Read the model definition and answer for the solid it produces. Units are mm, in the model's axes. A direction names the side the tool comes from. Coordinates: 2 decimals unless noted, no trailing zeros. Order: outer loops, then holes, each group sorted by start corner. A loop starts at its lowest first (then second) coordinate and runs counter-clockwise, first axis right, second up. Notation, with made-up numbers: (52, 52.5) - (85, 52.5) arc R24 ccw to (85, 79.5) - close; hole circle Ø3 at (24, -15.5). An arc over 180 degrees is marked (long way). Use one line per item in the form item = value.
```python
from build123d import *

# Parameters (mm, degrees)
ESBO_O1_W                = 100
ESBO_O1_H                = 100
RESSALTO_EXTRUS_O1_DEPTH = 5
ESBO_O2_R                = 7.5
ESBO_O2_R_2              = 5
RESSALTO_EXTRUS_O2_DEPTH = 60


with BuildPart() as part:
    # Esboço1 → Ressalto-extrusão1 (new body)
    with BuildSketch(Plane(origin=(0, 0, 0), x_dir=(1, 0, 0), z_dir=(0, 1, 0))):
        Rectangle(ESBO_O1_W, ESBO_O1_H)
    extrude(amount=-RESSALTO_EXTRUS_O1_DEPTH)

    # Esboço2 → Ressalto-extrusão2 (add)
    with BuildSketch(Plane(origin=(0, 0, 0), x_dir=(1, 0, 0), z_dir=(0, 1, 0))):
        with Locations(Location((0, 0, 0), (0, 0, 270))):
            Circle(ESBO_O2_R)
        with Locations(Location((0, 0, 0), (0, 0, 270))):
            Circle(ESBO_O2_R_2, mode=Mode.SUBTRACT)
    extrude(amount=RESSALTO_EXTRUS_O2_DEPTH)


solid = part.part
```
(1) Section A-A, the plane z = 0 is taken. Write down the section's boundary in (x, y).
Answer list:
outline = (-50, -5) - (50, -5) - (50, 0) - (7.5, 0) - (7.5, 60) - (5, 60) - (5, 0) - (-5, 0) - (-5, 60) - (-7.5, 60) - (-7.5, 0) - (-50, 0) - close
(2) Section D-D, the plane z = -15 is taken. Write down the section's boundary in (x, y), then the cut area to 3 significant figures.
Answer list:
outline = (-50, -5) - (50, -5) - (50, 0) - (-50, 0) - close
area = 500 mm2
(3) Given pin 1 Ø5 at (x, z) = (10.5, 10.5) entering from +Y; pin 2 Ø6 at (x, y) = (0.5, 43.5) entering from -Z, each flat-ended and moving along its own axis, determine where each tip first touches the part or whether it passes through.
Answer list:
pin_1 = 0
pin_2 = -7.5
(4) Section B-B, the plane x = 0 is taken. Write down the section's boundary in (y, z).
Answer list:
outline = (-5, -50) - (0, -50) - (0, -7.5) - (60, -7.5) - (60, -5) - (0, -5) - (0, 5) - (60, 5) - (60, 7.5) - (0, 7.5) - (0, 50) - (-5, 50) - close
(5) The mould has two halves that part along X. Classify faces 3 (the flat face through (0, 0, 0)), 4 (the cylindrical face through (-4.88, 29.58, -1.08)), 5 (the flat face through (-50, -2, 1)), 6 (the flat face through (-1, -2, 50)): +X half, -X half, draft (parallel to the pull), parting line (faces both ways), or undercut.
Answer list:
face_3 = undercut
face_4 = undercut
face_5 = -X half
face_6 = draft
(6) Straight lines are drawn through the part: L1, parallel to X at y = 35, z = 0; L2, parallel to Y at x = 40, z = 37.5. For each, find the intervals that lie inside material, in ascending order.
Answer list:
L1 = -7.5 to -5, 5 to 7.5
L2 = -5 to 0
(7) Section C-C, the plane y = 22 is taken. Write down the section's boundary in (x, z), then the cut area to 3 significant figures.
Answer list:
outline = circle Ø15 at (0, 0); hole circle Ø10 at (0, 0)
area = 98.2 mm2
(8) Which of the six approach directions +Z, -Z, +X, -X, +Y, -Y give full straight-line access (tool end or side, diameter ignored) to faces 1 (the cylindrical face through (0.33, 29.58, -7.493)), 2 (the flat face through (-1, -5, -1))?
Answer list:
face_1 = +Y
face_2 = +Z, -Z, +X, -X, -Y
